Verification items for the finished model (mm, model axes). Face numbers are marked on the shaded views. A direction names the side the tool comes from. Coordinates: 2 decimals unless noted, no trailing zeros. Order: outer loops, then holes, each group sorted by start corner. A loop starts at its lowest first (then second) coordinate and runs counter-clockwise, first axis right, second up. Notation, with made-up numbers: (29.5, 14) - (80.5, 14) arc R29 ccw to (80.5, 48) - close; hole circle Ø5 at (36.5, 84.5). An arc over 180 degrees is marked (long way). Answer as CSV lines item,"result". Start each with the question number.
1. Mould release check, pull along Y, two halves, no side actions. Record for the marked faces 1, 2 and 3: pulls with the +Y half, pulls with the -Y half, needs draft (parallel to the pull), parting line crosses it, or undercut.
2. Section check C-C (y = -10). Record the cut outline in (x, z), and give its area (3 significant figures).
3. Set-up check for the marked faces 4 and 5: record each of +Z, -Z, +X, -X, +Y, -Y from which the full face is reachable in a straight line by a thin tool's end or side.
4. Section check B-B (z = 203). Record the cut outline in (x, y).
5. Material ranges on L1, parallel to Z at x = 45, y = -34 (3 decimals); L2, parallel to X at y = -33.25, z = 75 (3 decimals); L3, parallel to X at y = -36.5, z = 165 (3 decimals), recorded low to high. Write a range as [from, to].
6. Section check D-D (x = -25). Record the cut outline in (y, z), and give its area (3 significant figures).
7. Section check A-A (y = 41). Record the cut outline in (x, z), and give its area (3 significant figures).
8. Go/stop test with flat-tipped pins: pin 1 (8 mm diameter, centred on x = -45, y = -40, fed in from +Z); pin 2 (3 mm diameter, centred on x = 46, z = 165.5, fed in from +Y); pin 3 (6 mm diameter, centred on x = -68, z = 94, fed in from +Y). Record where each tip stops, or that it passes through.
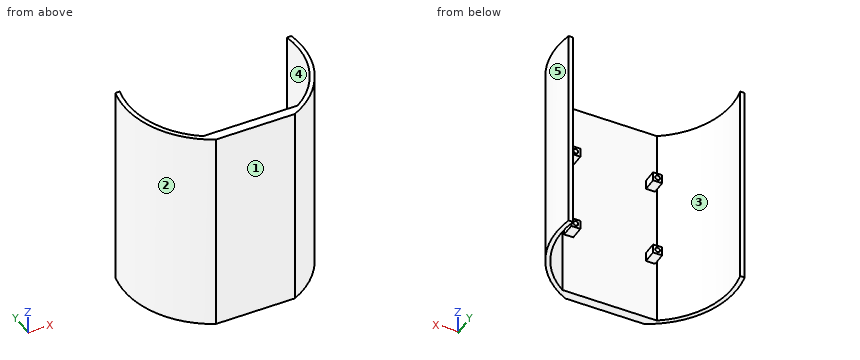
Autodesk Inventor part; units mm, degrees
ref_plane "YZ Plane" through (0, 0, 0) normal (1, 0, 0) x (0, 1, 0)
ref_plane "XZ Plane" through (0, 0, 0) normal (0, 1, 0) x (-1, 0, 0)
ref_plane "XY Plane" through (0, 0, 0) normal (0, 0, 1) x (1, 0, 0)
sketch "Sketch1" plane through (0, 0, 0) normal (0, 0, 1) x (1, 0, 0)
  arc A0 (-96.8589, 55) -> (-43.4971, -55) centre (0, 34.0439) ccw
  line L0 (-43.4971, -55) -> (43.4971, -55)
  arc A1 (43.4971, -55) -> (96.8589, 55) centre (0, 34.0439) ccw
  line L1 (96.8589, 55) -> (91.8589, 55)
  arc A2 (51.9882, -44.5338) -> (91.8589, 55) centre (0, 34.0439) ccw
  arc A3 (-91.8589, 55) -> (-51.9882, -44.5338) centre (0, 34.0439) ccw
  line L2 (-91.8589, 55) -> (-96.8589, 55)
  line L3 (51.9882, -44.5338) -> (-51.9882, -44.5338)
  point P0 (0, 0)
extrude "Extrusion1" add sketch "Sketch1" along normal blind 230
sketch "Sketch2" plane through (-43.4971, -44.5338, 0) normal (0, 1, 0) x (1, 0, 0)
  circle A0 centre (-1.5029, -75) radius 1.6 construction
  circle A1 centre (-1.5029, -165) radius 1.6 construction
  circle A2 centre (88.4971, -75) radius 1.6 construction
  circle A3 centre (88.4971, -165) radius 1.6 construction
  line L0 (-6.5029, -70) -> (-6.5029, -170) construction
  line L1 (-6.5029, -170) -> (93.4971, -170) construction
  line L2 (93.4971, -170) -> (93.4971, -70) construction
  line L3 (93.4971, -70) -> (-6.5029, -70) construction
  line L4 (86.9943, 0) -> (0, 0) construction
  line L5 (0, 0) -> (0, -230) construction
  line L6 (86.9943, -230) -> (0, -230) construction
  line L7 (86.9943, 0) -> (86.9943, -230) construction
  line L8 (-6.5029, -80) -> (3.4971, -80)
  line L9 (3.4971, -80) -> (3.4971, -70)
  line L10 (3.4971, -70) -> (-6.5029, -70)
  line L11 (-6.5029, -70) -> (-6.5029, -80)
  line L12 (-6.5029, -80) -> (3.4971, -70) construction
  line L13 (3.4971, -80) -> (-6.5029, -70) construction
  line L14 (83.4971, -80) -> (93.4971, -80)
  line L15 (93.4971, -80) -> (93.4971, -70)
  line L16 (93.4971, -70) -> (83.4971, -70)
  line L17 (83.4971, -70) -> (83.4971, -80)
  line L18 (83.4971, -80) -> (93.4971, -70) construction
  line L19 (93.4971, -80) -> (83.4971, -70) construction
  line L20 (3.4971, -170) -> (-6.5029, -170)
  line L21 (-6.5029, -170) -> (-6.5029, -160)
  line L22 (-6.5029, -160) -> (3.4971, -160)
  line L23 (3.4971, -160) -> (3.4971, -170)
  line L24 (3.4971, -170) -> (-6.5029, -160) construction
  line L25 (-6.5029, -170) -> (3.4971, -160) construction
  line L26 (83.4971, -170) -> (93.4971, -170)
  line L27 (93.4971, -170) -> (93.4971, -160)
  line L28 (93.4971, -160) -> (83.4971, -160)
  line L29 (83.4971, -160) -> (83.4971, -170)
  line L30 (83.4971, -170) -> (93.4971, -160) construction
  line L31 (93.4971, -170) -> (83.4971, -160) construction
  point P0 (43.4971, 0)
  dimension "d2" = 10
  dimension "d3" = 10
  dimension "d4" = 10
  dimension "d5" = 10
  dimension "d6" = 10
  dimension "d7" = 10
  dimension "d8" = 10
  dimension "d9" = 10
extrude "Extrusion2" add sketch "Sketch2" along normal blind 15
sketch "Sketch3" plane through (-43.4971, -29.5338, 0) normal (0, 1, 0) x (1, 0, 0)
  circle A0 centre (-1.5029, -75) radius 1.6 construction
  circle A1 centre (-1.5029, -165) radius 1.6 construction
  circle A2 centre (88.4971, -75) radius 1.6 construction
  circle A3 centre (88.4971, -165) radius 1.6 construction
  line L0 (-6.5029, -70) -> (-6.5029, -170) construction
  line L1 (-6.5029, -170) -> (93.4971, -170) construction
  line L2 (93.4971, -170) -> (93.4971, -70) construction
  line L3 (93.4971, -70) -> (-6.5029, -70) construction
  circle A4 centre (-1.5029, -75) radius 2.665
  circle A5 centre (88.4971, -75) radius 2.665
  circle A6 centre (88.4971, -165) radius 2.665
  circle A7 centre (-1.5029, -165) radius 2.665
  point P0 (43.4971, 0)
  dimension "d12" = 5.33
  dimension "d13" = 5.33
  dimension "d14" = 5.33
  dimension "d15" = 5.33
extrude "Extrusion3" cut sketch "Sketch3" against normal blind 11.5
sketch "Sketch4" plane through (0, 0, 0) normal (0, 0, -1) x (-1, 0, 0)
  arc A0 (43.4971, -55) -> (96.8589, 55) centre (0, 34.0439) ccw construction
  line L0 (43.4971, -55) -> (-43.4971, -55) construction
  arc A1 (-96.8589, 55) -> (-43.4971, -55) centre (0, 34.0439) ccw construction
  line L1 (-96.8589, 55) -> (-91.8589, 55) construction
  arc A2 (-91.8589, 55) -> (-51.9882, -44.5338) centre (0, 34.0439) ccw construction
  line L2 (-51.9882, -44.5338) -> (51.9882, -44.5338) construction
  arc A3 (51.9882, -44.5338) -> (91.8589, 55) centre (0, 34.0439) ccw construction
  line L3 (91.8589, 55) -> (96.8589, 55) construction
  arc A4 (43.4971, -55) -> (96.8589, 55) centre (0, 34.0439) ccw construction
  line L4 (43.4971, -55) -> (-43.4971, -55) construction
  arc A5 (-96.8589, 55) -> (-43.4971, -55) centre (0, 34.0439) ccw construction
  line L5 (-96.8589, 55) -> (-91.8589, 55) construction
  arc A6 (-91.8589, 55) -> (-51.9882, -44.5338) centre (0, 34.0439) ccw construction
  arc A7 (51.9882, -44.5338) -> (91.8589, 55) centre (0, 34.0439) ccw construction
  line L6 (91.8589, 55) -> (96.8589, 55) construction
  line L7 (-51.9882, -44.5338) -> (51.9882, -44.5338)
  line L8 (47.665, -29.5338) -> (47.665, -41.0338)
  line L9 (-43.4971, -49.5338) -> (43.4971, -49.5338)
  arc A8 (-51.9882, -44.5338) -> (-43.4971, -49.5338) centre (0, 34.0439) ccw
  arc A9 (43.4971, -49.5338) -> (51.9882, -44.5338) centre (0, 34.0439) ccw
  arc A10 (43.4971, -49.5338) -> (91.8589, 55) centre (0, 34.0439) ccw
  line L10 (-51.9882, -44.5338) -> (51.9882, -44.5338)
  point P0 (0, 0)
extrude "Extrusion4" add sketch "Sketch4" against normal blind 30
properties part number "BackInsertV1_3DPrint"
Evaluation:
1,face 1,"pulls with the -Y half"
1,face 2,"parting line crosses it"
1,face 3,"undercut"
2,outline,"(-88.77, 0) - (-83.29, 0) - (-83.29, 230) - (-88.77, 230) - close; (83.29, 0) - (88.77, 0) - (88.77, 230) - (83.29, 230) - close"
2,area,"2,520 mm²"
3,face 4,"+Z, -Z"
3,face 5,"+Z, -Z, +X"
4,outline,"(-96.86, 55) arc R99.1 ccw to (-43.5, -55) - (43.5, -55) arc R99.1 ccw to (96.86, 55) - (91.86, 55) arc R94.22 cw to (51.99, -44.53) - (-51.99, -44.53) arc R94.22 cw to (-91.86, 55) - close"
5,L1,"z = [70, 72.335], [77.665, 80], [160, 162.335], [167.665, 170]"
5,L2,"x = [-72.748, -65.945], [-50, -47.665], [-42.335, -40], [40, 42.335], [47.665, 50], [65.945, 72.749]"
5,L3,"x = [-69.601, -62.456], [-50, -47.665], [-42.335, -40], [40, 42.335], [47.665, 50], [62.456, 69.602]"
6,outline,"(-55, 0) - (-44.53, 0) - (-44.53, 230) - (-55, 230) - close"
6,area,"2,410 mm²"
7,outline,"(-98.86, 0) - (-93.96, 0) - (-93.96, 230) - (-98.86, 230) - close; (93.96, 0) - (98.86, 0) - (98.86, 230) - (93.96, 230) - close"
7,area,"2,250 mm²"
8,pin 1,"stops at z = 170"
8,pin 2,"stops at y = -41.03"
8,pin 3,"stops at y = -27.89"
